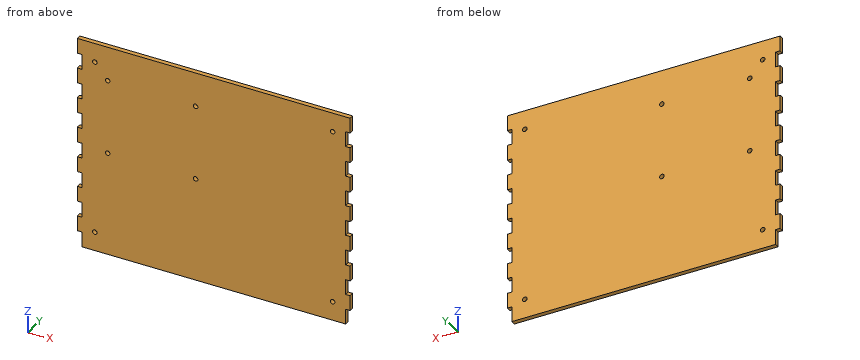
```python
from build123d import *

# Parameters (mm, degrees)
ESQUISSE1_W             = 180
ESQUISSE1_H             = 140
ESQUISSE1_R             = 1.5
BOSS_EXTRU_1_DEPTH      = 3
ENL_V_MAT_EXTRU_1_REACH = 5
ESQUISSE2_W             = 3
ESQUISSE2_H             = 10


with BuildPart() as part:
    # Esquisse1 → Boss.-Extru.1 (new body)
    with BuildSketch(Plane(origin=(0, 0, 0), x_dir=(1, 0, 0), z_dir=(0, 1, 0))):
        Rectangle(ESQUISSE1_W, ESQUISSE1_H)
        with Locations((-78.45, 57.48)):
            Circle(ESQUISSE1_R, mode=Mode.SUBTRACT)
        with Locations((78.45, 57.48)):
            Circle(ESQUISSE1_R, mode=Mode.SUBTRACT)
        with Locations((78.45, -57.48)):
            Circle(ESQUISSE1_R, mode=Mode.SUBTRACT)
        with Locations((-78.45, -57.48)):
            Circle(ESQUISSE1_R, mode=Mode.SUBTRACT)
        with Locations((-69.95, 1.57626837)):
            Circle(ESQUISSE1_R, mode=Mode.SUBTRACT)
        with Locations((-11.95, 1.57626837)):
            Circle(ESQUISSE1_R, mode=Mode.SUBTRACT)
        with Locations((-69.95, -47.42373163)):
            Circle(ESQUISSE1_R, mode=Mode.SUBTRACT)
        with Locations((-11.95, -47.42373163)):
            Circle(ESQUISSE1_R, mode=Mode.SUBTRACT)
    extrude(amount=BOSS_EXTRU_1_DEPTH)

    # Esquisse2 → Enlèv. mat.-Extru.1 (cut, up to next)
    with BuildSketch(Plane(origin=(0, 3, 0), x_dir=(1, 0, 0), z_dir=(0, 1, 0)), mode=Mode.PRIVATE) as enl_v_mat_extru_1_sk1:
        with Locations((-88.5, 45)):
            Rectangle(ESQUISSE2_W, ESQUISSE2_H)
    enl_v_mat_extru_1_tool1 = extrude(enl_v_mat_extru_1_sk1.sketch, amount=-ENL_V_MAT_EXTRU_1_REACH, mode=Mode.PRIVATE) & part.part
    add(enl_v_mat_extru_1_tool1.solids().sort_by_distance((-88.5, 3, -45))[0], mode=Mode.SUBTRACT)
    # Esquisse2 → Enlèv. mat.-Extru.1 (cut, up to next)
    with BuildSketch(Plane(origin=(0, 3, 0), x_dir=(1, 0, 0), z_dir=(0, 1, 0)), mode=Mode.PRIVATE) as enl_v_mat_extru_1_sk2:
        with Locations((-88.5, 65)):
            Rectangle(ESQUISSE2_W, ESQUISSE2_H)
    enl_v_mat_extru_1_tool2 = extrude(enl_v_mat_extru_1_sk2.sketch, amount=-ENL_V_MAT_EXTRU_1_REACH, mode=Mode.PRIVATE) & part.part
    add(enl_v_mat_extru_1_tool2.solids().sort_by_distance((-88.5, 3, -65))[0], mode=Mode.SUBTRACT)
    # Esquisse2 → Enlèv. mat.-Extru.1 (cut, up to next)
    with BuildSketch(Plane(origin=(0, 3, 0), x_dir=(1, 0, 0), z_dir=(0, 1, 0)), mode=Mode.PRIVATE) as enl_v_mat_extru_1_sk3:
        with Locations((-88.5, 25)):
            Rectangle(ESQUISSE2_W, ESQUISSE2_H)
    enl_v_mat_extru_1_tool3 = extrude(enl_v_mat_extru_1_sk3.sketch, amount=-ENL_V_MAT_EXTRU_1_REACH, mode=Mode.PRIVATE) & part.part
    add(enl_v_mat_extru_1_tool3.solids().sort_by_distance((-88.5, 3, -25))[0], mode=Mode.SUBTRACT)
    # Esquisse2 → Enlèv. mat.-Extru.1 (cut, up to next)
    with BuildSketch(Plane(origin=(0, 3, 0), x_dir=(1, 0, 0), z_dir=(0, 1, 0)), mode=Mode.PRIVATE) as enl_v_mat_extru_1_sk4:
        with Locations((-88.5, 5)):
            Rectangle(ESQUISSE2_W, ESQUISSE2_H)
    enl_v_mat_extru_1_tool4 = extrude(enl_v_mat_extru_1_sk4.sketch, amount=-ENL_V_MAT_EXTRU_1_REACH, mode=Mode.PRIVATE) & part.part
    add(enl_v_mat_extru_1_tool4.solids().sort_by_distance((-88.5, 3, -5))[0], mode=Mode.SUBTRACT)
    # Esquisse2 → Enlèv. mat.-Extru.1 (cut, up to next)
    with BuildSketch(Plane(origin=(0, 3, 0), x_dir=(1, 0, 0), z_dir=(0, 1, 0)), mode=Mode.PRIVATE) as enl_v_mat_extru_1_sk5:
        with Locations((-88.5, -15)):
            Rectangle(ESQUISSE2_W, ESQUISSE2_H)
    enl_v_mat_extru_1_tool5 = extrude(enl_v_mat_extru_1_sk5.sketch, amount=-ENL_V_MAT_EXTRU_1_REACH, mode=Mode.PRIVATE) & part.part
    add(enl_v_mat_extru_1_tool5.solids().sort_by_distance((-88.5, 3, 15))[0], mode=Mode.SUBTRACT)
    # Esquisse2 → Enlèv. mat.-Extru.1 (cut, up to next)
    with BuildSketch(Plane(origin=(0, 3, 0), x_dir=(1, 0, 0), z_dir=(0, 1, 0)), mode=Mode.PRIVATE) as enl_v_mat_extru_1_sk6:
        with Locations((-88.5, -35)):
            Rectangle(ESQUISSE2_W, ESQUISSE2_H)
    enl_v_mat_extru_1_tool6 = extrude(enl_v_mat_extru_1_sk6.sketch, amount=-ENL_V_MAT_EXTRU_1_REACH, mode=Mode.PRIVATE) & part.part
    add(enl_v_mat_extru_1_tool6.solids().sort_by_distance((-88.5, 3, 35))[0], mode=Mode.SUBTRACT)
    # Esquisse2 → Enlèv. mat.-Extru.1 (cut, up to next)
    with BuildSketch(Plane(origin=(0, 3, 0), x_dir=(1, 0, 0), z_dir=(0, 1, 0)), mode=Mode.PRIVATE) as enl_v_mat_extru_1_sk7:
        with Locations((-88.5, -55)):
            Rectangle(ESQUISSE2_W, ESQUISSE2_H)
    enl_v_mat_extru_1_tool7 = extrude(enl_v_mat_extru_1_sk7.sketch, amount=-ENL_V_MAT_EXTRU_1_REACH, mode=Mode.PRIVATE) & part.part
    add(enl_v_mat_extru_1_tool7.solids().sort_by_distance((-88.5, 3, 55))[0], mode=Mode.SUBTRACT)
    # Esquisse2 → Enlèv. mat.-Extru.1 (cut, up to next)
    with BuildSketch(Plane(origin=(0, 3, 0), x_dir=(1, 0, 0), z_dir=(0, 1, 0)), mode=Mode.PRIVATE) as enl_v_mat_extru_1_sk8:
        with Locations((88.5, -55)):
            Rectangle(ESQUISSE2_W, ESQUISSE2_H)
    enl_v_mat_extru_1_tool8 = extrude(enl_v_mat_extru_1_sk8.sketch, amount=-ENL_V_MAT_EXTRU_1_REACH, mode=Mode.PRIVATE) & part.part
    add(enl_v_mat_extru_1_tool8.solids().sort_by_distance((88.5, 3, 55))[0], mode=Mode.SUBTRACT)
    # Esquisse2 → Enlèv. mat.-Extru.1 (cut, up to next)
    with BuildSketch(Plane(origin=(0, 3, 0), x_dir=(1, 0, 0), z_dir=(0, 1, 0)), mode=Mode.PRIVATE) as enl_v_mat_extru_1_sk9:
        with Locations((88.5, -35)):
            Rectangle(ESQUISSE2_W, ESQUISSE2_H)
    enl_v_mat_extru_1_tool9 = extrude(enl_v_mat_extru_1_sk9.sketch, amount=-ENL_V_MAT_EXTRU_1_REACH, mode=Mode.PRIVATE) & part.part
    add(enl_v_mat_extru_1_tool9.solids().sort_by_distance((88.5, 3, 35))[0], mode=Mode.SUBTRACT)
    # Esquisse2 → Enlèv. mat.-Extru.1 (cut, up to next)
    with BuildSketch(Plane(origin=(0, 3, 0), x_dir=(1, 0, 0), z_dir=(0, 1, 0)), mode=Mode.PRIVATE) as enl_v_mat_extru_1_sk10:
        with Locations((88.5, -15)):
            Rectangle(ESQUISSE2_W, ESQUISSE2_H)
    enl_v_mat_extru_1_tool10 = extrude(enl_v_mat_extru_1_sk10.sketch, amount=-ENL_V_MAT_EXTRU_1_REACH, mode=Mode.PRIVATE) & part.part
    add(enl_v_mat_extru_1_tool10.solids().sort_by_distance((88.5, 3, 15))[0], mode=Mode.SUBTRACT)
    # Esquisse2 → Enlèv. mat.-Extru.1 (cut, up to next)
    with BuildSketch(Plane(origin=(0, 3, 0), x_dir=(1, 0, 0), z_dir=(0, 1, 0)), mode=Mode.PRIVATE) as enl_v_mat_extru_1_sk11:
        with Locations((88.5, 5)):
            Rectangle(ESQUISSE2_W, ESQUISSE2_H)
    enl_v_mat_extru_1_tool11 = extrude(enl_v_mat_extru_1_sk11.sketch, amount=-ENL_V_MAT_EXTRU_1_REACH, mode=Mode.PRIVATE) & part.part
    add(enl_v_mat_extru_1_tool11.solids().sort_by_distance((88.5, 3, -5))[0], mode=Mode.SUBTRACT)
    # Esquisse2 → Enlèv. mat.-Extru.1 (cut, up to next)
    with BuildSketch(Plane(origin=(0, 3, 0), x_dir=(1, 0, 0), z_dir=(0, 1, 0)), mode=Mode.PRIVATE) as enl_v_mat_extru_1_sk12:
        with Locations((88.5, 25)):
            Rectangle(ESQUISSE2_W, ESQUISSE2_H)
    enl_v_mat_extru_1_tool12 = extrude(enl_v_mat_extru_1_sk12.sketch, amount=-ENL_V_MAT_EXTRU_1_REACH, mode=Mode.PRIVATE) & part.part
    add(enl_v_mat_extru_1_tool12.solids().sort_by_distance((88.5, 3, -25))[0], mode=Mode.SUBTRACT)
    # Esquisse2 → Enlèv. mat.-Extru.1 (cut, up to next)
    with BuildSketch(Plane(origin=(0, 3, 0), x_dir=(1, 0, 0), z_dir=(0, 1, 0)), mode=Mode.PRIVATE) as enl_v_mat_extru_1_sk13:
        with Locations((88.5, 45)):
            Rectangle(ESQUISSE2_W, ESQUISSE2_H)
    enl_v_mat_extru_1_tool13 = extrude(enl_v_mat_extru_1_sk13.sketch, amount=-ENL_V_MAT_EXTRU_1_REACH, mode=Mode.PRIVATE) & part.part
    add(enl_v_mat_extru_1_tool13.solids().sort_by_distance((88.5, 3, -45))[0], mode=Mode.SUBTRACT)
    # Esquisse2 → Enlèv. mat.-Extru.1 (cut, up to next)
    with BuildSketch(Plane(origin=(0, 3, 0), x_dir=(1, 0, 0), z_dir=(0, 1, 0)), mode=Mode.PRIVATE) as enl_v_mat_extru_1_sk14:
        with Locations((88.5, 65)):
            Rectangle(ESQUISSE2_W, ESQUISSE2_H)
    enl_v_mat_extru_1_tool14 = extrude(enl_v_mat_extru_1_sk14.sketch, amount=-ENL_V_MAT_EXTRU_1_REACH, mode=Mode.PRIVATE) & part.part
    add(enl_v_mat_extru_1_tool14.solids().sort_by_distance((88.5, 3, -65))[0], mode=Mode.SUBTRACT)


solid = part.part
```
Could you check a few things on this model? Use its own coordinates, in mm. Give positions to 0.01 mm unless a question says otherwise; leave off trailing zeros. Loops run counter-clockwise (first coordinate to the right, second up) from the corner with the lowest first, then second, coordinate; pieces in that order, holes last. Notation, with made-up numbers: (-25, 84) - (-9, 84) arc R20 ccw to (-9, 108) - close; hole circle Ø5 at (-18.75, -9.75). An arc over 180 degrees is marked (long way). Use one line per item in the form item = value.
1. I want a section at B-B (y = 2.1). Give the number of separate pieces and of enclosed holes in the cut face, and give its area (3 significant figures).
Response values:
separate_pieces = 1
enclosed_holes = 8
area = 24,700 mm²
2. I want a section at A-A (z = 16.5). Please give me the cut outline in (x, y), and give its area (3 significant figures).
Response values:
outline = (-87, 0) - (87, 0) - (87, 3) - (-87, 3) - close
area = 522 mm²
3. I'm going to push flat-ended pins straight in: pin 1 Ø0.9 at (x, y) = (-88, 2) entering from -Z; pin 2 Ø0.9 at (y, z) = (1.5, 34) entering from +X; pin 3 Ø1.5 at (y, z) = (1, -66.5) entering from -X. Where does each tip first touch, or does it pass through?
Response values:
pin_1 = -60
pin_2 = 87
pin_3 = -87
4. I need wall thicknesses on probe 1 along Z at (x, y) = (-69.95, 0.8); probe 2 along Z at (x, y) = (-78.45, 0.85); probe 3 along X at (y, z) = (0.85, -57.48). Which ranges of each line are inside material? Lowest first, please.
Response values:
probe_1 = -70 to -3.08, -0.08 to 45.92, 48.92 to 70
probe_2 = -70 to -58.98, -55.98 to 55.98, 58.98 to 70
probe_3 = -90 to -79.95, -76.95 to 76.95, 79.95 to 90
